Answer from the drawing. Dimensions are ordinates in mm from the lowest x, y and z of the part. Coordinates: 2 decimals unless noted, no trailing zeros. Write each loop counter-clockwise with the first axis right and the second up, starting at its lowest first coordinate (ties: lowest second). Pieces come first, ordered by that corner, then holes. Notation, with made-up numbers: (-15, 23) -> (-9, 23) arc R22 cw to (-9, 55) -> close; hole circle Ø7 at (45, -3.5). An arc over 180 degrees is marked (long way). Return JSON: item names as keys, results as strings.
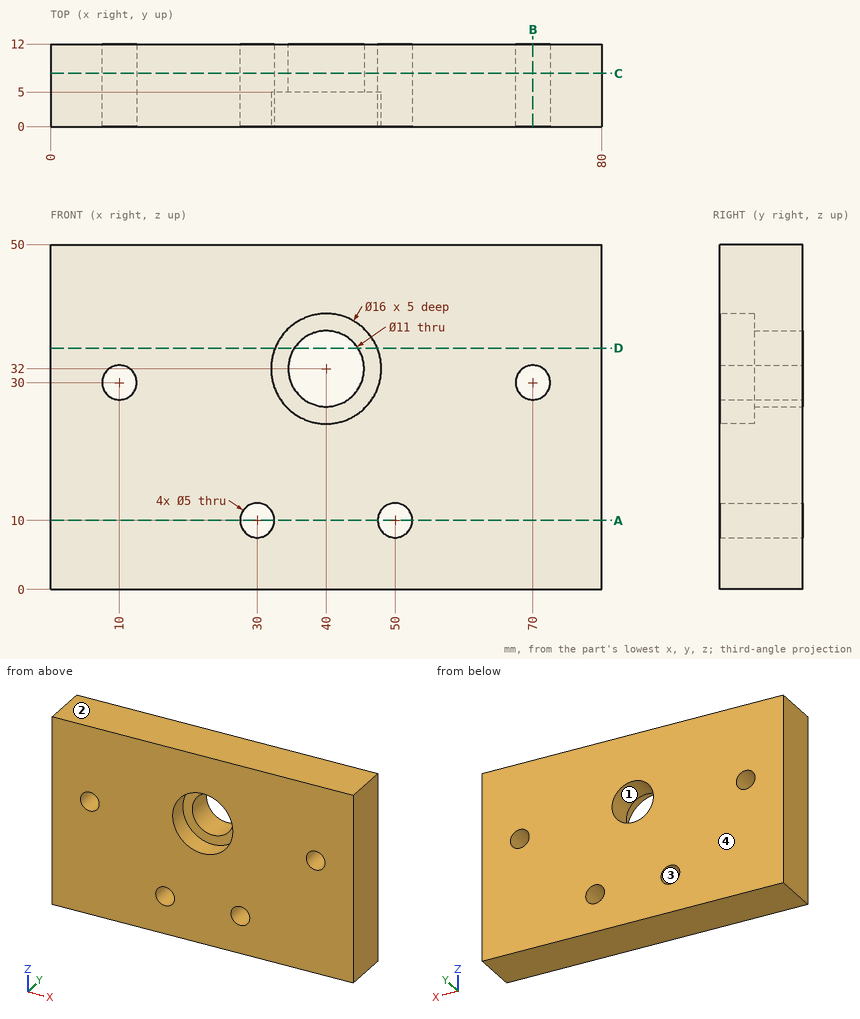
1. The part is cut by section A-A (z = 10). Determine the outline of the cut face in (x, y), then the cut area to 3 significant figures.
Taken from the geometry:
{"outline": "(0, 0) -> (27.5, 0) -> (27.5, 12) -> (0, 12) -> close; (32.5, 0) -> (47.5, 0) -> (47.5, 12) -> (32.5, 12) -> close; (52.5, 0) -> (80, 0) -> (80, 12) -> (52.5, 12) -> close", "area": "840 mm2"}
2. The part is cut by section D-D (z = 35). Determine the outline of the cut face in (x, y), then the cut area to 3 significant figures.
Taken from the geometry:
{"outline": "(0, 0) -> (32.58, 0) -> (32.58, 5) -> (35.39, 5) -> (35.39, 12) -> (0, 12) -> close; (44.61, 5) -> (47.42, 5) -> (47.42, 0) -> (80, 0) -> (80, 12) -> (44.61, 12) -> close", "area": "821 mm2"}
3. For a pull along Z with two mould halves and no side action, classify the marked faces 1, 2, 3 and 4 as +Z half, -Z half, draft (parallel to the pull), parting line (faces both ways), or undercut.
Taken from the geometry:
{"face 1": "undercut", "face 2": "+Z half", "face 3": "undercut", "face 4": "draft"}
4. Consider L1, parallel to Z at x = 40, y = 9.25; L2, parallel to Z at x = 40, y = 1.75; L3, parallel to X at y = 3.75, z = 38.5. Determine where each line is inside the solid, lowest interval first.
Taken from the geometry:
{"L1": "z = 0 to 26.5, 37.5 to 50", "L2": "z = 0 to 24, 40 to 50", "L3": "x = 0 to 35.34, 44.66 to 80"}
5. Flat-ended cylindrical pins translate along their axes: pin 1 Ø5 at (x, y) = (16.5, 10.5) entering from -Z; pin 2 Ø9.5 at (x, z) = (40, 32) entering from +Y. Find the tip coordinate at first contact, or state that the pin passes through.
Taken from the geometry:
{"pin 1": "stops at z = 0", "pin 2": "passes through"}
6. The part is cut by section B-B (x = 70). Determine the outline of the cut face in (y, z).
Taken from the geometry:
{"outline": "(0, 0) -> (12, 0) -> (12, 27.5) -> (0, 27.5) -> close; (0, 32.5) -> (12, 32.5) -> (12, 50) -> (0, 50) -> close"}
7. The part is cut by section C-C (y = 7.75). Determine the outline of the cut face in (x, z), then the cut area to 3 significant figures.
Taken from the geometry:
{"outline": "(0, 0) -> (80, 0) -> (80, 50) -> (0, 50) -> close; hole circle Ø5 at (10, 30); hole circle Ø5 at (30, 10); hole circle Ø11 at (40, 32); hole circle Ø5 at (50, 10); hole circle Ø5 at (70, 30)", "area": "3,830 mm2"}
